For this review, take the finished solid that the model builds, in its own axes (mm). A direction names the side the tool comes from. Round coordinates to 2 decimals unless told otherwise and drop trailing zeros. Write each loop counter-clockwise with the first axis right and the second up, starting at its lowest first coordinate (ties: lowest second). Pieces come first, ordered by that corner, then holes.
from build123d import *

# Parameters (mm, degrees)
SKETCH1_W           = 220
SKETCH1_H           = 30
BOSS_EXTRUDE1_DEPTH = 30
SKETCH2_R           = 10.1
CUT_EXTRUDE1_DEPTH  = 30
SKETCH3_R           = 10.1
CUT_EXTRUDE2_DEPTH  = 30
FILLET1_R           = 8
FILLET2_R           = 8
FILLET4_R           = 7
SCALE1_SCALE        = 0.5


with BuildPart() as part:
    # Sketch1 → Boss-Extrude1 (new body)
    with BuildSketch(Plane(origin=(0, 0, 0), x_dir=(0, 0, -1), z_dir=(1, 0, 0))):
        with BuildLine():
            Line((-122.679491924, 10), (-10, 10))
            Line((-10, 10), (-10, 25))
            Line((-10, 25), (235, 25))
            Line((235, 25), (235, 10))
            Line((235, 10), (250, 10))
            ThreePointArc((250, 10), (287.320508076, 0), (250, -10))
            Line((250, -10), (235, -10))
            Line((235, -10), (235, -25))
            Line((235, -25), (-10, -25))
            Line((-10, -25), (-10, -10))
            Line((-10, -10), (-122.679491924, -10))
            ThreePointArc((-122.679491924, -10), (-160, 0), (-122.679491924, 10))
        make_face()
        with Locations((110, 0)):
            Rectangle(SKETCH1_W, SKETCH1_H, mode=Mode.SUBTRACT)
    extrude(amount=BOSS_EXTRUDE1_DEPTH)

    # Sketch2 → Cut-Extrude1 (cut)
    with BuildSketch(Plane(origin=(0, 0, 0), x_dir=(0, 0, -1), z_dir=(1, 0, 0))):
        with Locations((-140, 0)):
            Circle(SKETCH2_R)
    extrude(amount=CUT_EXTRUDE1_DEPTH, mode=Mode.SUBTRACT)

    # Sketch3 → Cut-Extrude2 (cut)
    with BuildSketch(Plane.ZY):
        with Locations((-267.320508076, 0)):
            Circle(SKETCH3_R)
    extrude(amount=-CUT_EXTRUDE2_DEPTH, mode=Mode.SUBTRACT)

    # Fillet1
    fillet1_edges = [part.edges().sort_by_distance(p)[0] for p in [
        (0, -10, 66.339745962),
        (0, 0, 160),
        (0, 10, 66.339745962),
        (30, 10, 66.339745962),
        (30, 0, 160),
        (15, -10, 122.679491924),
        (15, 10, 122.679491924),
        (30, -10, 66.339745962),
    ]]
    fillet(fillet1_edges, radius=FILLET1_R)

    # Fillet2
    fillet2_edges = [part.edges().sort_by_distance(p)[0] for p in [
        (0, 10, -242.5),
        (0, 0, -287.320508076),
        (0, -10, -242.5),
        (15, 10, -250),
        (15, -10, -250),
        (30, -10, -242.5),
        (30, 0, -287.320508076),
        (30, 10, -242.5),
    ]]
    fillet(fillet2_edges, radius=FILLET2_R)

    # Fillet4
    fillet4_edges = [part.edges().sort_by_distance(p)[0] for p in [
        (15, -25, 10),
        (30, -25, -112.5),
        (15, -25, -235),
        (0, -25, -112.5),
        (15, 25, -235),
        (30, 25, -112.5),
        (15, 25, 10),
        (0, 25, -112.5),
        (30, 13.5, -235),
        (0, 13.5, -235),
        (0, 13.5, 10),
        (30, -13.5, 10),
    ]]
    fillet(fillet4_edges, radius=FILLET4_R)


with BuildPart() as part_1:
    # Scale1: scaled about (0, 0, 0)
    add(part.part.scale(SCALE1_SCALE))


solid = part_1.part
(1) We need section B-B, the plane x = 7.25. Give the boundary of the cut face in (y, z).
Geometry check:
outline: (-12.5, -114) arc R3.5 ccw to (-9, -117.5) - (-5, -117.5) - (-5, -122.94) arc R4 cw to (-6.43, -126) arc R10 ccw (long way) to (6.43, -126) arc R4 cw to (5, -122.94) - (5, -117.5) - (9, -117.5) arc R3.5 ccw to (12.5, -114) - (12.5, 1.5) arc R3.5 ccw to (9, 5) - (5, 5) - (5, 59.28) arc R4 cw to (6.43, 62.34) arc R10 ccw (long way) to (-6.43, 62.34) arc R4 cw to (-5, 59.28) - (-5, 5) - (-9, 5) arc R3.5 ccw to (-12.5, 1.5) - close; hole (-7.5, -110) - (7.5, -110) - (7.5, 0) - (-7.5, 0) - close; hole circle Ø10.1 at (0, -133.66); hole circle Ø10.1 at (0, 70)
(2) For faces 1 (the face through (9.33, 11.5, 3.95)), 2 (the face through (1.203, 3.859, 29.984)), 3 (the face through (14.389, -5.945, 3.476)), 4 (the face through (7, -5, -120)), list the 3-axis set-ups (+Z, -Z, +X, -X, +Y, -Y) from which the entire face can be reached by the end or side of a thin tool; tool diameter is ignored.
Geometry check:
face 1: +X, -X, +Y
face 2: -X, +Y
face 3: +X, -Y
face 4: +X, -X, -Y
(3) For pin 1 Ø3 at (x, y) = (7, 7.5) entering from -Z; pin 2 Ø2.5 at (x, y) = (5, -6) entering from -Z; pin 3 Ø1.5 at (x, y) = (2.5, 9) entering from +Z, all flat-tipped, find the tip position at first contact; note any pin that passes through.
Geometry check:
pin 1: stops at z = -141.66
pin 2: stops at z = -142.46
pin 3: stops at z = 75.22
(4) For line 1 along Y through (x, z) = (7, -42); line 2 along Z through (x, y) = (12.5, 8.75); line 3 along Y through (x, z) = (5.5, 70), list the stretches that pass through material, from the lowest coordinate up.
Geometry check:
line 1: y = -12.5 to -7.5, 7.5 to 12.5
line 2: z = -137.87 to -129.45, -117.35 to 5, 65.79 to 74.21
line 3: y = -10 to -5.05, 5.05 to 10
(5) Mouldability with a two-part tool opening along Z and no side actions: class faces 5 (the face through (7.451, 0.342, -143.654)), 6 (the face through (7, 0, 80)), 7 (the face through (14, -11.45, -57.17)) as pulls with the +Z half, pulls with the -Z half, needs draft (parallel to the pull), parting line crosses it, or undercut.
Geometry check:
face 5: undercut
face 6: undercut
face 7: needs draft
(6) We need section C-C, the plane z = 46. Give the boundary of the cut face in (x, y), and give its area (3 significant figures).
Geometry check:
outline: (0, -1) arc R4 ccw to (4, -5) - (11, -5) arc R4 ccw to (15, -1) - (15, 1) arc R4 ccw to (11, 5) - (4, 5) arc R4 ccw to (0, 1) - close
area: 136 mm2
(7) We need section A-A, the plane z = -4.5. Give the boundary of the cut face in (x, y), and give its area (3 significant figures).
Geometry check:
outline: (0, -9) arc R3.5 ccw to (3.5, -12.5) - (11.5, -12.5) arc R3.5 ccw to (15, -9) - (15, -7.5) - (0, -7.5) - close; (0, 7.5) - (15, 7.5) - (15, 9) arc R3.5 ccw to (11.5, 12.5) - (3.5, 12.5) arc R3.5 ccw to (0, 9) - close
area: 139 mm2
